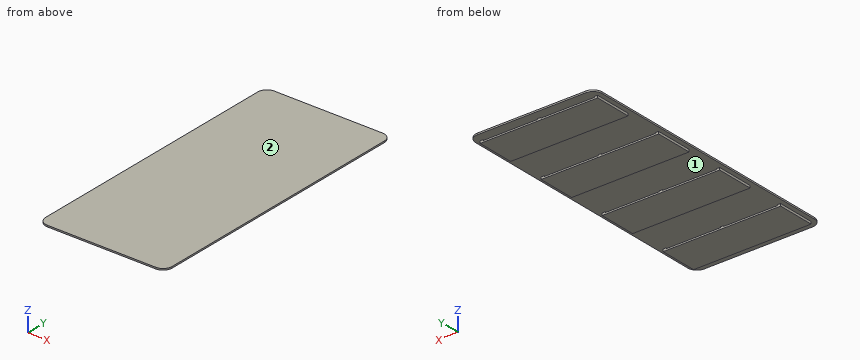
from build123d import *

# Parameters (mm, degrees)
PAD044_DEPTH            = 1
PAD043_DEPTH            = 25
LINEARPATTERN_COUNT     = 4
LINEARPATTERN_PITCH     = 50
BODY028_PLACEMENT_ANGLE = 180


with BuildPart() as part:
    # Sketch114 → Pad044 (new body)
    with BuildSketch(Plane.XY):
        with BuildLine():
            Line((-42, 147), (-42, -27))
            ThreePointArc((-42, -27), (-40.242641, -31.242641), (-36, -33))
            Line((-36, -33), (36, -33))
            ThreePointArc((36, -33), (40.242641, -31.242641), (42, -27))
            Line((42, -27), (42, 147))
            ThreePointArc((42, 147), (40.242641, 151.242641), (36, 153))
            Line((36, 153), (-36, 153))
            ThreePointArc((-36, 153), (-40.242641, 151.242641), (-42, 147))
        make_face()
    extrude(amount=PAD044_DEPTH)

    # Sketch113 → Pad043 (join)
    with BuildSketch(Plane.XZ.offset(28)):
        Polygon((-39, 2.5), (39, 2.5), (39, 0), (38, 0), (37, 0), (37, 1.5), (1, 1.5), (1, 0), (0, 0), (-1, 0), (-1, 1.5), (-37, 1.5), (-37, 0), (-38, 0), (-39, 0), align=None)
    pad043 = extrude(amount=-PAD043_DEPTH)

    # LinearPattern: Pad043 ×4
    with Locations(*[(0, i * LINEARPATTERN_PITCH, 0) for i in range(1, LINEARPATTERN_COUNT)]):
        add(pad043)


with BuildPart() as part_1:
    # Body028 placement: moved
    add(part.part.moved(Location((0, -59, 31))).rotate(Axis((0, -59, 31), (0, 1, 0)), BODY028_PLACEMENT_ANGLE))


solid = part_1.part
Input: part model. Units: mm. Frame: model coordinates. Face numbers are marked on the shaded views. Coordinates: 2 decimals unless noted, no trailing zeros. Loops run counter-clockwise (first coordinate to the right, second up) from the corner with the lowest first, then second, coordinate; pieces in that order, holes last.
Q1. Material intervals for line 1 (X direction, y = 14, z = 29.8); line 2 (Y direction, x = 17, z = 29.1); line 3 (Z direction, x = -8, y = -17), sorted ascending.
Q2. Draft query along X for the marked faces 1 and 2. Return one class per face: +X half, -X half, draft (parallel to the pull), parting line (faces both ways), or undercut.
Q3. Contact query for flat-ended pins moving along their axis: pin 1 (0.8 mm diameter, centred on y = 23, z = 29.5, fed in from +X); pin 2 (1.2 mm diameter, centred on y = -79, z = 29, fed in from -X); pin 3 (0.8 mm diameter, centred on x = 18.5, z = 29, fed in from -Y). Output: stop coordinate, or through.
Q4. Cut plane B-B (y = -74.5). Output: boundary loops of the cut face in (x, z).
Q5. Cut plane A-A (x = 31.5). Output: boundary loops of the cut face in (y, z).
Q6. Cut plane C-C (y = 51.5). Output: boundary loops of the cut face in (x, z).
Working result:
1. line 1: x = -39 to -37, -1 to 1, 37 to 39
1. line 2: y = -87 to -62, -37 to -12, 13 to 38, 63 to 88
1. line 3: z = 28.5 to 29.5, 30 to 31
2. face 1: undercut
2. face 2: draft
3. pin 1: stops at x = 39
3. pin 2: stops at x = -39
3. pin 3: stops at y = -87
4. outline: (-42, 30) - (-39, 30) - (-39, 28.5) - (39, 28.5) - (39, 30) - (42, 30) - (42, 31) - (-42, 31) - close; hole (-37, 29.5) - (-1, 29.5) - (-1, 30) - (-37, 30) - close; hole (1, 29.5) - (37, 29.5) - (37, 30) - (1, 30) - close
5. outline: (-92, 30) - (94, 30) - (94, 31) - (-92, 31) - close; (-87, 28.5) - (-62, 28.5) - (-62, 29.5) - (-87, 29.5) - close; (-37, 28.5) - (-12, 28.5) - (-12, 29.5) - (-37, 29.5) - close; (13, 28.5) - (38, 28.5) - (38, 29.5) - (13, 29.5) - close; (63, 28.5) - (88, 28.5) - (88, 29.5) - (63, 29.5) - close
6. outline: (-42, 30) - (42, 30) - (42, 31) - (-42, 31) - close
